Verification items for this drawing (mm, ordinates from the low corner). A direction names the side the tool comes from. Round coordinates to 2 decimals unless told otherwise and drop trailing zeros. Write each loop counter-clockwise with the first axis right and the second up, starting at its lowest first coordinate (ties: lowest second). Pieces come first, ordered by that corner, then holes. Notation, with made-up numbers: (63.25, -23.5) - (69.25, -23.5) arc R25 cw to (69.25, -5.5) - close; hole circle Ø6 at (-38.75, 70.25). An arc over 180 degrees is marked (long way). One line per question, with ' | ' between items. Start each with the question number.
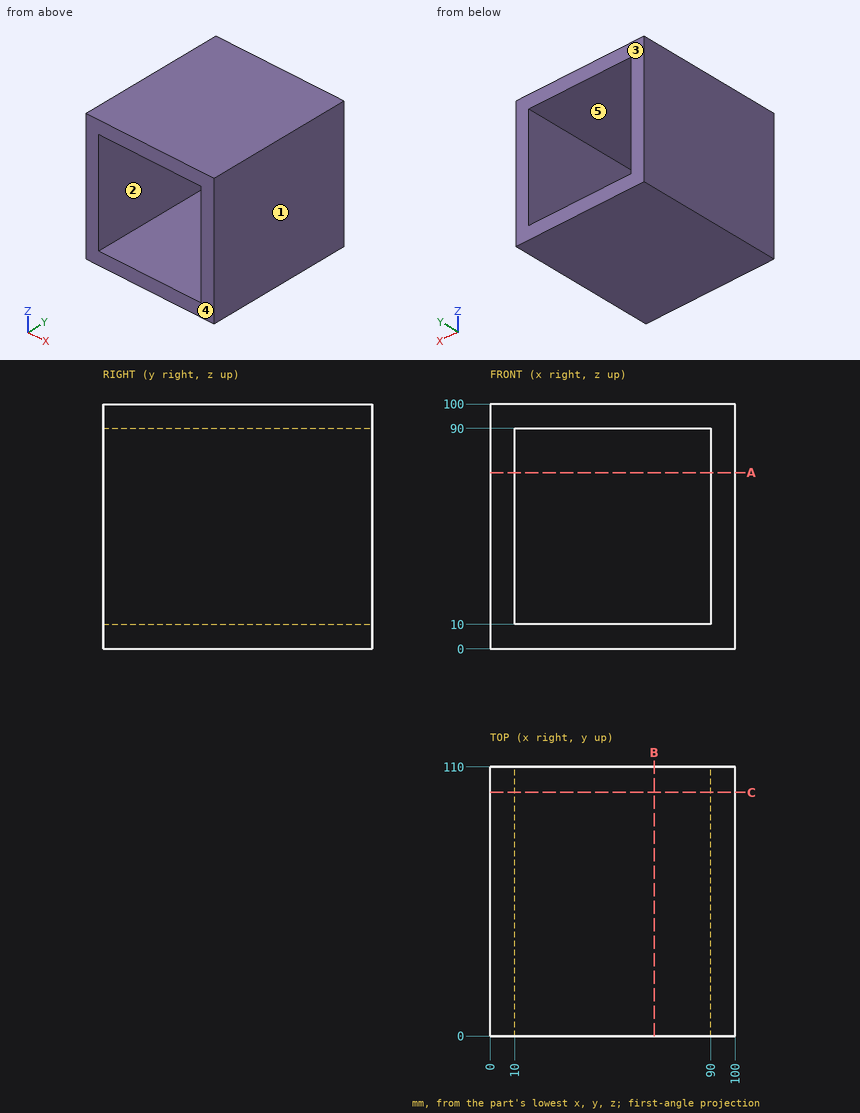
Q1. Set-up check for the marked faces 4 and 5: record each of +Z, -Z, +X, -X, +Y, -Y from which the full face is reachable in a straight line by a thin tool's end or side.
Q2. Draft check along X on the marked faces 1, 2 and 3. Enter one of: pulls with the +X half, pulls with the -X half, needs draft (parallel to the pull), parting line crosses it, or undercut.
Q3. Section check B-B, the plane x = 67. Record the cut outline in (y, z), then the cut area to 3 significant figures.
Q4. Thickness scan on line 1 (X direction, y = 12.5, z = 35.5). Record the ranges inside material, lowest first.
Q5. Section check C-C, the plane y = 99.5. Record the cut outline in (x, z), then the cut area to 3 significant figures.
Q6. Section check A-A, the plane z = 72. Record the cut outline in (x, y).
Result sheet:
1) face 4: +Z, -Z, +X, -X, -Y | face 5: +Y, -Y
2) face 1: pulls with the +X half | face 2: undercut | face 3: needs draft
3) outline: (0, 0) - (110, 0) - (110, 10) - (0, 10) - close; (0, 90) - (110, 90) - (110, 100) - (0, 100) - close | area: 2,200 mm²
4) line 1: 0 to 10, 90 to 100
5) outline: (0, 0) - (100, 0) - (100, 100) - (0, 100) - close; hole (10, 10) - (90, 10) - (90, 90) - (10, 90) - close | area: 3,600 mm²
6) outline: (0, 0) - (10, 0) - (10, 110) - (0, 110) - close; (90, 0) - (100, 0) - (100, 110) - (90, 110) - close
